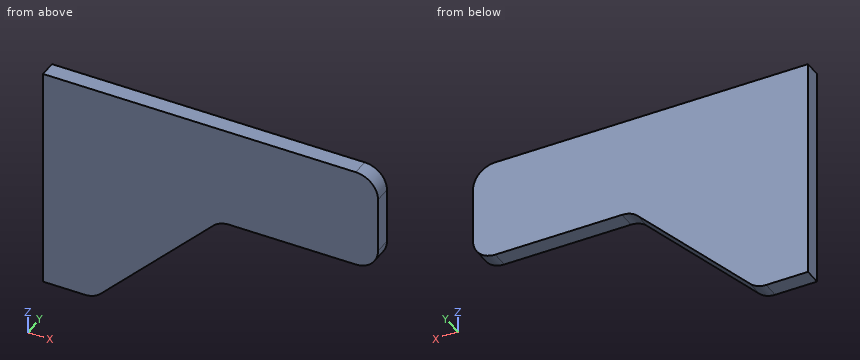
from build123d import *

# Parameters (mm, degrees)
F1_DEPTH = 6


with BuildPart() as f1:
    # F0 (on Front) → F1 (new body)
    with BuildSketch(Plane.XZ):
        with BuildLine():
            ThreePointArc((15, -81), (18.061467, -80.391036), (20.656854, -78.656854))
            Line((20.656854, -78.656854), (60.970563, -38.343146))
            ThreePointArc((60.970563, -38.343146), (63.56595, -36.608964), (66.627417, -36))
            Line((66.627417, -36), (112, -36))
            ThreePointArc((112, -36), (117.656854, -33.656854), (120, -28))
            Line((120, -28), (120, -8))
            ThreePointArc((120, -8), (117.656854, -2.343146), (112, 0))
            Line((112, 0), (0, 0))
            Line((0, 0), (0, -81))
            Line((0, -81), (15, -81))
        make_face()
    extrude(amount=F1_DEPTH)


solid = f1.part
CAD build for the part. Positions are in the model's coordinates, mm. Round coordinates to 2 decimals unless told otherwise and drop trailing zeros. Loops run counter-clockwise (first coordinate to the right, second up) from the corner with the lowest first, then second, coordinate; pieces in that order, holes last.
(1) Drop flat-ended pins along their axis: pin 1 (1 mm diameter, centred on y = -3.5, z = -34, fed in from +X); pin 2 (8 mm diameter, centred on x = 37, z = -33.5, fed in from +Y); pin 3 (1.8 mm diameter, centred on x = 83.5, y = -4, fed in from -Z); pin 4 (2 mm diameter, centred on y = -1.5, z = -41, fed in from +X). Give the stop position or say it passes through.
(2) Wall check: line 1 along Z through (x, y) = (112.5, -1.95); line 2 along Z through (x, y) = (61, -0.9); line 3 along X through (y, z) = (-0.3, -49). Give the ranges that are in metal, low to high.
(3) Cut at C-C (z = -72). Give the cut face in (x, y).
(4) Cut at B-B (x = 105.5). Give the cut face in (y, z), plus the area to 3 significant figures.
(5) Cut at A-A (y = -4.1). Give the cut face in (x, z).
Findings below:
1. pin 1: stops at x = 117.81
1. pin 2: stops at y = 0
1. pin 3: stops at z = -36
1. pin 4: stops at x = 59.31
2. line 1: z = -35.98 to -0.02
2. line 2: z = -38.31 to 0
2. line 3: x = 0 to 50.31
3. outline: (0, -6) - (27.31, -6) - (27.31, 0) - (0, 0) - close
4. outline: (-6, -36) - (0, -36) - (0, 0) - (-6, 0) - close
4. area: 216 mm2
5. outline: (0, -81) - (15, -81) arc R8 ccw to (20.66, -78.66) - (60.97, -38.34) arc R8 cw to (66.63, -36) - (112, -36) arc R8 ccw to (120, -28) - (120, -8) arc R8 ccw to (112, 0) - (0, 0) - close
